Can you work these out from the model? Positions are in its coordinate system, mm. Face numbers are marked on the shaded views. Round coordinates to 2 decimals unless told otherwise and drop trailing zeros. Loops run counter-clockwise (first coordinate to the right, second up) from the corner with the lowest first, then second, coordinate; pieces in that order, holes last.
(1) Will these pins go through, and if not, where does the flat tip stop? pin 1 Ø0.8 at (y, z) = (3, 60.5) entering from +X; pin 2 Ø1.1 at (y, z) = (3.5, 125) entering from +X; pin 3 Ø1.1 at (x, y) = (1.5, 3.5) entering from +Z.
(2) I want a section at B-B on y = 3.4. Give the number of separate pieces and of enclosed holes in the cut face, plus the area to 3 significant figures.
(3) I want a section at C-C on x = 25. Write out the boundary of the cut face in (y, z), plus the area to 3 significant figures.
(4) I want a section at A-A on z = 33.5. Write out the boundary of the cut face in (x, y), plus the area to 3 significant figures.
(5) If I drill on line 1 along Z through (x, y) = (20, 2.85); line 2 along Z through (x, y) = (-9, 5.6); line 3 along Z through (x, y) = (13.5, 4.75), over which ranges is the centre line in solid material (lowest first)?
(6) Thinking about a two-plate mould opening in Y: for the marked faces 1 and 2, which applies, released by +Y, released by -Y, zero draft, split by the parting line, or undercut?
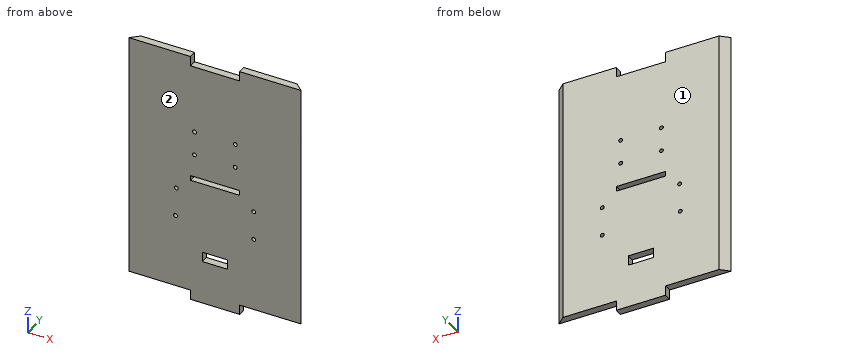
from build123d import *

# Parameters (mm, degrees)
BOSS_EXTRUDE1_DEPTH = 127
SKETCH3_W           = 25.4
SKETCH3_H           = 5.08
CUT_EXTRUDE1_DEPTH  = 135.591199998
SKETCH4_W           = 25.4
SKETCH4_H           = 5.08
BOSS_EXTRUDE3_DEPTH = 3.81
SKETCH5_R           = 1
SKETCH5_R_2         = 0.999998
SKETCH5_W           = 13
SKETCH5_H           = 5.08
SKETCH5_W_2         = 25.4
SKETCH5_H_2         = 2.54
CUT_EXTRUDE2_DEPTH  = 135.591199998


with BuildPart() as part:
    # Sketch1 → Boss-Extrude1 (new body)
    with BuildSketch(Plane.XY):
        Polygon((-40.203883769, 5.937788296), (40.203883769, 5.937788296), (44.399042974, 2.127788296), (-44.399042974, 2.127788296), align=None)
    extrude(amount=BOSS_EXTRUDE1_DEPTH)

    # Sketch3 → Cut-Extrude1 (cut, through all)
    with BuildSketch(Plane.XZ.offset(-2.127788296)):
        with Locations((0, 124.46)):
            Rectangle(SKETCH3_W, SKETCH3_H)
    extrude(amount=-CUT_EXTRUDE1_DEPTH, mode=Mode.SUBTRACT)

    # Sketch4 → Boss-Extrude3 (add)
    with BuildSketch(Plane.XZ.offset(-2.127788296)):
        with Locations((0, -2.504739817)):
            Rectangle(SKETCH4_W, SKETCH4_H)
    extrude(amount=-BOSS_EXTRUDE3_DEPTH)

    # Sketch5 → Cut-Extrude2 (cut, through all)
    with BuildSketch(Plane(origin=(0, 2.127788296, 0), x_dir=(-1, 0, 0), z_dir=(0, -1, 0))):
        with Locations(Location((-19.96, -38.1, 0), (0, 0, 90))):
            Circle(SKETCH5_R)
        with Locations(Location((20.313021022, -38.1, 0), (0, 0, 90))):
            Circle(SKETCH5_R)
        with Locations(Location((19.96, -53.142840099, 0), (0, 0, 90))):
            Circle(SKETCH5_R)
        with Locations(Location((-19.96, -53.142840099, 0), (0, 0, 90))):
            Circle(SKETCH5_R)
        with Locations(Location((-10.44215584, -74.203260183, 0), (0, 0, 90))):
            Circle(SKETCH5_R)
        with Locations(Location((-10.44215584, -86.649260183, 0), (0, 0, 90))):
            Circle(SKETCH5_R)
        with Locations(Location((10.55784416, -74.203260183, 0), (0, 0, 90))):
            Circle(SKETCH5_R)
        with Locations(Location((10.55784416, -86.649260183, 0), (0, 0, 90))):
            Circle(SKETCH5_R)
        with Locations((-93.931058926, -72.649749874)):
            Circle(SKETCH5_R_2)
        with Locations((-93.931058926, -85.149749874)):
            Circle(SKETCH5_R)
        with Locations((-72.931058926, -72.649749874)):
            Circle(SKETCH5_R)
        with Locations((-72.931058926, -85.149749874)):
            Circle(SKETCH5_R)
        with Locations((-93.904836904, 5.641456719)):
            Circle(SKETCH5_R)
        with Locations((-53.184836904, 5.641456719)):
            Circle(SKETCH5_R)
        with Locations((-53.184836904, -9.358543281)):
            Circle(SKETCH5_R)
        with Locations((-93.904836904, -9.358543281)):
            Circle(SKETCH5_R)
        with Locations((0, -20.02)):
            Rectangle(SKETCH5_W, SKETCH5_H)
        with Locations((0, -60.995260183)):
            Rectangle(SKETCH5_W_2, SKETCH5_H_2)
    extrude(amount=-CUT_EXTRUDE2_DEPTH, mode=Mode.SUBTRACT)


solid = part.part
Filled sheet:
1. pin 1: stops at x = 43.88
1. pin 2: stops at x = 43.49
1. pin 3: stops at z = 121.92
2. separate pieces: 1
2. enclosed holes: 10
2. area: 10,800 mm2
3. outline: (2.13, 0) - (5.94, 0) - (5.94, 127) - (2.13, 127) - close
3. area: 484 mm2
4. outline: (-44.4, 2.13) - (44.4, 2.13) - (40.2, 5.94) - (-40.2, 5.94) - close
4. area: 322 mm2
5. line 1: z = 0 to 37.1, 39.1 to 52.14, 54.14 to 127
5. line 2: z = -5.04 to 59.73, 62.27 to 121.92
5. line 3: z = 0 to 127
6. face 1: released by +Y
6. face 2: released by -Y
